from build123d import *

# Parameters (mm, degrees)
SKETCH1_W           = 43.18
SKETCH1_H           = 17.78
SKETCH1_R           = 0.889
BOSS_EXTRUDE1_DEPTH = 1.57
SKETCH2_W           = 5
SKETCH2_H           = 3.75
BOSS_EXTRUDE2_DEPTH = 2.5


with BuildPart() as part:
    # Sketch1 → Boss-Extrude1 (new body)
    with BuildSketch(Plane(origin=(0, 0, 0), x_dir=(1, 0, 0), z_dir=(0, 1, 0))):
        with Locations((-17.071162791, 9.812965116)):
            Rectangle(SKETCH1_W, SKETCH1_H)
        with Locations(Location((-37.391162791, 17.432965116, 0), (0, 0, 270))):
            Circle(SKETCH1_R, mode=Mode.SUBTRACT)
        with Locations(Location((-37.391162791, 2.192965116, 0), (0, 0, 270))):
            Circle(SKETCH1_R, mode=Mode.SUBTRACT)
        with Locations(Location((3.248837209, 2.192965116, 0), (0, 0, 270))):
            Circle(SKETCH1_R, mode=Mode.SUBTRACT)
        with Locations(Location((3.248837209, 17.432965116, 0), (0, 0, 270))):
            Circle(SKETCH1_R, mode=Mode.SUBTRACT)
    extrude(amount=BOSS_EXTRUDE1_DEPTH)

    # Sketch2 → Boss-Extrude2 (add)
    with BuildSketch(Plane(origin=(0, 1.57, 0), x_dir=(1, 0, 0), z_dir=(0, 1, 0))):
        with Locations((-36.161162791, 11.687965116)):
            Rectangle(SKETCH2_W, SKETCH2_H)
        with Locations((-36.161162791, 7.937965116)):
            Rectangle(SKETCH2_W, SKETCH2_H)
    extrude(amount=BOSS_EXTRUDE2_DEPTH)


solid = part.part
For this review, take the finished solid that the model builds, in its own axes (mm). A direction names the side the tool comes from. Round coordinates to 2 decimals unless told otherwise and drop trailing zeros. Order: outer loops, then holes, each group sorted by start corner. A loop starts at its lowest first (then second) coordinate and runs counter-clockwise, first axis right, second up. Notation, with made-up numbers: M 29,23 L 80,23 A22 ccw 80,39 Z; hole C -14.75,-35 d2. An arc over 180 degrees is marked long. Use a Markdown table: item, result. Add a question column.
Item 1: Add section A-A, the plane z = -10.5. Give the boundary of the cut face in (x, y), then the cut area to 3 significant figures.
Item 2: Add section C-C, the plane x = -7.5. Give the boundary of the cut face in (y, z), then the cut area to 3 significant figures.
Item 3: Tool access review of faces 4 (the cylindrical face through (-36.51, 0.77, -2.31)), 5 (the flat face through (-33.661, 3, -10)), 6 (the flat face through (-36, 3, -13.563)): name each direction out of +Z, -Z, +X, -X, +Y, -Y from which nothing blocks a thin tool from reaching the whole face with its end or side.
Item 4: Insertion check: pin 1 (1.2 mm diameter, centred on y = 2.5, z = -10.5, fed in from +X); pin 2 (2 mm diameter, centred on x = -17.5, z = -14, fed in from +Y); pin 3 (1.5 mm diameter, centred on y = 3.5, z = -4.5, fed in from -X); pin 4 (2 mm diameter, centred on x = -35, y = 3, fed in from +Z). Each pin has a flat end and moves straight along its axis. Give the tip position at first contact, or say it passes through.
Item 5: Add section B-B, the plane y = 3.6. Give the boundary of the cut face in (x, z).
Item 6: Mouldability with a two-part tool opening along X and no side actions: class faces 1 (the flat face through (-36, 3, -6.063)), 2 (the cylindrical face through (2.38, 0.77, -2.39)), 3 (the flat face through (4.519, 1, -10)) as released by +X, released by -X, zero draft, split by the parting line, or undercut.
Item 7: To check wall thickness, follow line 1 along X through (y, z) = (2.25, -7); line 2 along Y through (x, z) = (-29, -5.5). State the ranges of each line that lie inside material, in increasing order.
Geometry results:
| question | item | result |
|---|---|---|
| 1 | outline | M -38.66,0 L 4.52,0 L 4.52,1.57 L -33.66,1.57 L -33.66,4.07 L -38.66,4.07 Z |
| 1 | area | 80.3 mm² |
| 2 | outline | M 0,-18.7 L 1.57,-18.7 L 1.57,-0.92 L 0,-0.92 Z |
| 2 | area | 27.9 mm² |
| 3 | face 4 | +Y, -Y |
| 3 | face 5 | +Z, -Z, +X, +Y |
| 3 | face 6 | -Z, +X, -X, +Y |
| 4 | pin 1 | stops at x = -33.66 |
| 4 | pin 2 | stops at y = 1.57 |
| 4 | pin 3 | passes through |
| 4 | pin 4 | stops at z = -6.06 |
| 5 | outline | M -38.66,-13.56 L -33.66,-13.56 L -33.66,-6.06 L -38.66,-6.06 Z |
| 6 | face 1 | zero draft |
| 6 | face 2 | undercut |
| 6 | face 3 | released by +X |
| 7 | line 1 | x = -38.66 to -33.66 |
| 7 | line 2 | y = 0 to 1.57 |
